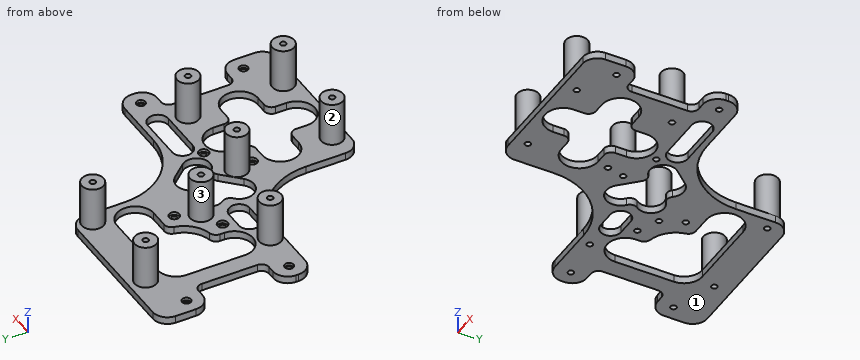
from build123d import *

# Parameters (mm, degrees)
SKICA1_W                 = 202
SKICA1_H                 = 202
P_IDAT_VYSUNUT_M1_DEPTH  = 5
ODEBRAT_VYSUNUT_M1_DEPTH = 10
SKICA3_R                 = 2
ODEBRAT_VYSUNUT_M2_DEPTH = 143.923056223
SKICA4_R                 = 3
ODEBRAT_VYSUNUT_M3_DEPTH = 2
SKICA6_R                 = 7.5
P_IDAT_VYSUNUT_M2_DEPTH  = 30
SKICA7_R                 = 2
ODEBRAT_VYSUNUT_M4_DEPTH = 148.061211745
SKICA9_R                 = 3.5
ODEBRAT_VYSUNUT_M6_DEPTH = 2
SKICA11_R                = 2
ODEBRAT_VYSUNUT_M7_DEPTH = 146.95204692
SKICA13_W                = 112
SKICA13_H                = 8
SKICA13_W_2              = 20
SKICA13_H_2              = 48
ODEBRAT_VYSUNUT_M8_DEPTH = 146.95204692
SKICA14_W                = 20
SKICA14_H                = 48
ODEBRAT_VYSUNUT_M9_DEPTH = 141.534693226
ZAOBLIT1_R               = 5
ZAOBLIT2_R               = 10


with BuildPart() as part:
    # Skica1 → Přidat vysunutím1 (new body)
    with BuildSketch(Plane.XY):
        Rectangle(SKICA1_W, SKICA1_H)
    extrude(amount=P_IDAT_VYSUNUT_M1_DEPTH)

    # Skica2 → Odebrat vysunutím1 (cut)
    with BuildSketch(Plane.XY.offset(5)):
        with BuildLine():
            Line((11, 56), (11, 101))
            Line((11, 101), (101, 101))
            Line((101, 101), (101, 11))
            Line((101, 11), (56, 11))
            ThreePointArc((56, 11), (24.180194847, 24.180194847), (11, 56))
        make_face()
        with BuildLine():
            Line((-56, -11), (-101, -11))
            Line((-101, -11), (-101, -101))
            Line((-101, -101), (-11, -101))
            Line((-11, -101), (-11, -56))
            ThreePointArc((-11, -56), (-24.180194847, -24.180194847), (-56, -11))
        make_face()
    extrude(amount=-ODEBRAT_VYSUNUT_M1_DEPTH, mode=Mode.SUBTRACT)

    # Skica3 → Odebrat vysunutím2 (cut, through all)
    with BuildSketch(Plane.XY.offset(5)):
        with Locations((91, 0)):
            Circle(SKICA3_R)
        with Locations(Location((-91, 0, 0), (0, 0, 180))):
            Circle(SKICA3_R)
        with Locations((91, -70)):
            Circle(SKICA3_R)
        with Locations(Location((-91, 70, 0), (0, 0, 180))):
            Circle(SKICA3_R)
    extrude(amount=-ODEBRAT_VYSUNUT_M2_DEPTH, mode=Mode.SUBTRACT)

    # Skica4 → Odebrat vysunutím3 (cut)
    with BuildSketch(Plane.XY.offset(5)):
        with Locations((91, 0)):
            Circle(SKICA4_R)
        with Locations(Location((-91, 0, 0), (0, 0, 180))):
            Circle(SKICA4_R)
        with Locations((91, -70)):
            Circle(SKICA4_R)
        with Locations(Location((-91, 70, 0), (0, 0, 180))):
            Circle(SKICA4_R)
    extrude(amount=-ODEBRAT_VYSUNUT_M3_DEPTH, mode=Mode.SUBTRACT)

    # Skica6 → Přidat vysunutím2 (add)
    with BuildSketch(Plane.XY.offset(5)):
        with Locations((-61.5, 81.5)):
            Circle(SKICA6_R)
        with Locations(Location((-61.5, -3.5, 0), (0, 0, 270))):
            Circle(SKICA6_R)
        with Locations((3.5, 81.5)):
            Circle(SKICA6_R)
        with Locations((-21.5, 21.5)):
            Circle(SKICA6_R)
        with Locations((6.5, -18.5)):
            Circle(SKICA6_R)
        with Locations((6.5, -83.5)):
            Circle(SKICA6_R)
        with Locations(Location((66.5, -18.5, 0), (0, 0, 180))):
            Circle(SKICA6_R)
        with Locations(Location((66.5, -83.5, 0), (0, 0, 180))):
            Circle(SKICA6_R)
    extrude(amount=P_IDAT_VYSUNUT_M2_DEPTH)

    # Skica7 → Odebrat vysunutím4 (cut, through all)
    with BuildSketch(Plane.XY.offset(35)):
        with Locations((-21.5, 21.5)):
            Circle(SKICA7_R)
        with Locations((-61.5, 81.5)):
            Circle(SKICA7_R)
        with Locations((3.5, 81.5)):
            Circle(SKICA7_R)
        with Locations((-61.5, -3.5)):
            Circle(SKICA7_R)
        with Locations((6.5, -18.5)):
            Circle(SKICA7_R)
        with Locations((66.5, -18.5)):
            Circle(SKICA7_R)
        with Locations((6.5, -83.5)):
            Circle(SKICA7_R)
        with Locations((66.5, -83.5)):
            Circle(SKICA7_R)
    extrude(amount=-ODEBRAT_VYSUNUT_M4_DEPTH, mode=Mode.SUBTRACT)

    # Skica9 → Odebrat vysunutím6 (cut)
    with BuildSketch(Plane.XY.offset(5)):
        with Locations((-14.849242405, 36.062445841)):
            Circle(SKICA9_R)
        with Locations(Location((-36.062445841, 14.849242405, 0), (0, 0, 180))):
            Circle(SKICA9_R)
        with Locations(Location((30.405591591, -9.192388155, 0), (0, 0, 180))):
            Circle(SKICA9_R)
        with Locations((9.192388155, -30.405591591)):
            Circle(SKICA9_R)
    extrude(amount=-ODEBRAT_VYSUNUT_M6_DEPTH, mode=Mode.SUBTRACT)

    # Skica11 → Odebrat vysunutím7 (cut, through all)
    with BuildSketch(Plane.XY.offset(5)):
        with Locations((-36.062445841, 14.849242405)):
            Circle(SKICA11_R)
        with Locations((-14.849242405, 36.062445841)):
            Circle(SKICA11_R)
        with Locations((30.405591591, -9.192388155)):
            Circle(SKICA11_R)
        with Locations((9.192388155, -30.405591591)):
            Circle(SKICA11_R)
    extrude(amount=-ODEBRAT_VYSUNUT_M7_DEPTH, mode=Mode.SUBTRACT)

    # Skica13 → Odebrat vysunutím8 (cut, through all)
    with BuildSketch(Plane.XY.offset(5)):
        with BuildLine():
            Line((11.5, -38.5), (24, -38.5))
            Line((24, -38.5), (24, -26))
            ThreePointArc((24, -26), (36.5, -13.5), (49, -26))
            Line((49, -26), (49, -38.5))
            Line((49, -38.5), (61.5, -38.5))
            ThreePointArc((61.5, -38.5), (74, -51), (61.5, -63.5))
            Line((61.5, -63.5), (49, -63.5))
            Line((49, -63.5), (49, -76))
            ThreePointArc((49, -76), (36.5, -88.5), (24, -76))
            Line((24, -76), (24, -63.5))
            Line((24, -63.5), (11.5, -63.5))
            ThreePointArc((11.5, -63.5), (-1, -51), (11.5, -38.5))
        make_face()
        with Locations((-45, 97)):
            Rectangle(SKICA13_W, SKICA13_H)
        with Locations((45, -97)):
            Rectangle(SKICA13_W, SKICA13_H)
        with Locations((91, -35)):
            Rectangle(SKICA13_W_2, SKICA13_H_2)
        with BuildLine():
            Line((-3.535533906, -17.67766953), (11.313708499, -2.828427125))
            Line((11.313708499, -2.828427125), (13.435028843, -4.949747468))
            ThreePointArc((13.435028843, -4.949747468), (25.913285858, -5.189980909), (26.633630146, 7.269782907))
            Line((26.633630146, 7.269782907), (18.200646465, 17.112789878))
            ThreePointArc((18.200646465, 17.112789878), (10.441367607, 20.605236509), (2.80172418, 16.858312414))
            Line((2.80172418, 16.858312414), (0, 13.360531537))
            Line((0, 13.360531537), (-3.565848529, 16.216777939))
            ThreePointArc((-3.565848529, 16.216777939), (-15.556349186, 15.556349186), (-16.216777939, 3.565848529))
            Line((-16.216777939, 3.565848529), (-13.360531537, 0))
            Line((-13.360531537, 0), (-16.858312414, -2.80172418))
            ThreePointArc((-16.858312414, -2.80172418), (-18.055848259, -17.278087757), (-3.535533906, -17.67766953))
        make_face()
        with BuildLine():
            Line((70, 7), (40, 7))
            ThreePointArc((40, 7), (33, 0), (40, -7))
            Line((40, -7), (70, -7))
            ThreePointArc((70, -7), (77, 0), (70, 7))
        make_face()
        with BuildLine():
            Line((-42, -7), (-30, -7))
            ThreePointArc((-30, -7), (-23, 0), (-30, 7))
            Line((-30, 7), (-42, 7))
            ThreePointArc((-42, 7), (-49, 0), (-42, -7))
        make_face()
    extrude(amount=-ODEBRAT_VYSUNUT_M8_DEPTH, mode=Mode.SUBTRACT)

    # Skica14 → Odebrat vysunutím9 (cut, through all)
    with BuildSketch(Plane.XY.offset(5)):
        with Locations((-91, 35)):
            Rectangle(SKICA14_W, SKICA14_H)
        with BuildLine():
            Line((-69, 58), (-69, 18))
            ThreePointArc((-69, 18), (-56.5, 5.5), (-44, 18))
            Line((-44, 18), (-44, 25.5))
            ThreePointArc((-44, 25.5), (-29.857864376, 31.357864376), (-24, 45.5))
            Line((-24, 45.5), (-6.5, 45.5))
            ThreePointArc((-6.5, 45.5), (6, 58), (-6.5, 70.5))
            Line((-6.5, 70.5), (-56.5, 70.5))
            ThreePointArc((-56.5, 70.5), (-65.338834765, 66.838834765), (-69, 58))
        make_face()
    extrude(amount=-ODEBRAT_VYSUNUT_M9_DEPTH, mode=Mode.SUBTRACT)

    # Zaoblit1
    zaoblit1_edges = [part.edges().sort_by_distance(p)[0] for p in [
        (49, -38.5, 2.5),
        (24, -38.5, 2.5),
        (49, -63.5, 2.5),
        (24, -63.5, 2.5),
        (81, -59, 2.5),
        (81, -11, 2.5),
        (-24, 45.5, 2.5),
        (-44, 25.5, 2.5),
        (-81, 59, 2.5),
        (-81, 11, 2.5),
        (11.313708499, -2.828427125, 2.5),
        (-13.360531537, 0, 2.5),
        (0, 13.360531537, 2.5),
    ]]
    fillet(zaoblit1_edges, radius=ZAOBLIT1_R)

    # Zaoblit2
    zaoblit2_edges = [part.edges().sort_by_distance(p)[0] for p in [
        (101, 11, 2.5),
        (-101, 93, 2.5),
        (11, 93, 2.5),
        (101, -11, 2.5),
        (101, -59, 2.5),
        (-11, -93, 2.5),
        (101, -93, 2.5),
        (-101, -11, 2.5),
        (-101, 11, 2.5),
        (-101, 59, 2.5),
    ]]
    fillet(zaoblit2_edges, radius=ZAOBLIT2_R)


solid = part.part
The model under review builds one solid part; all positions refer to its coordinate system, in mm. Face numbers are marked on the shaded views. Round coordinates to 2 decimals unless told otherwise and drop trailing zeros. Order: outer loops, then holes, each group sorted by start corner. A loop starts at its lowest first (then second) coordinate and runs counter-clockwise, first axis right, second up. Notation, with made-up numbers: (79.5, 55) - (118.5, 55) arc R18 ccw to (118.5, 73) - close; hole circle Ø3 at (-16, 23). An arc over 180 degrees is marked (long way). Use one line per item in the form item = value.
Q1. To check wall thickness, follow line 1 (Y direction, x = -9, z = 3.5); line 2 (Y direction, x = 91, z = 1.2); line 3 (Y direction, x = 3.5, z = 18). State the ranges of each line that lie inside material, in increasing order.
Response values:
line_1 = -89 to -20.48, 18.19 to 45.5, 70.5 to 93
line_2 = -93 to -72, -68 to -59, -11 to -2, 2 to 11
line_3 = -90.37 to -76.63, -25.37 to -11.63, 74 to 79.5, 83.5 to 89
Q2. Mouldability with a two-part tool opening along X and no side actions: class the marked faces 1, 2 and 3 as pulls with the +X half, pulls with the -X half, needs draft (parallel to the pull), parting line crosses it, or undercut.
Response values:
face_1 = needs draft
face_2 = undercut
face_3 = parting line crosses it
Q3. Add section A-A on z = 11. Give the number of separate pieces and of enclosed holes in the cut face, then the cut area to 3 significant figures.
Response values:
separate_pieces = 8
enclosed_holes = 8
area = 1,310 mm^2
Q4. Add section B-B on y = -50. Give the boundary of the cut face in (x, z), then the cut area to 3 significant figures.
Response values:
outline = (-11.4, 0) - (-0.96, 0) - (-0.96, 5) - (-11.4, 5) - close; (73.96, 0) - (81, 0) - (81, 5) - (73.96, 5) - close
area = 87.4 mm^2
Q5. Clearance check with flat-ended pins moving along their axes: P1, Ø6.5, axis at x = -91.5, y = 69.5, coming from the +Z side; P2, Ø3.5, axis at x = -14.85, y = 36.06, coming from the -Z side; P3, Ø4, axis at x = 49, z = 3.5, coming from the +Y side; P4, Ø5.5, axis at y = -72.5, z = 2, coming from the -X side. State where each tip first meets the part, or that it passes through.
Response values:
P1 = 5
P2 = through
P3 = 11.91
P4 = -11
